from build123d import *

# Parameters (mm, degrees)
F0_W      = 25.4
F0_H      = 25.4
F1_DEPTH  = 27.94
F2_R      = 5.08
F3_R      = 5.08
F4_R      = 5.08
F5_R      = 5.08
F6_W      = 15.24
F6_H      = 7.62
F7_DEPTH  = 12.7
F8_R      = 2.54
F9_R      = 2.54
F10_R     = 2.54
F11_R     = 2.54
F12_R     = 3.175
F14_DEPTH = 9.525


with BuildPart() as f1:
    # F0 (on Front) → F1 (new body)
    with BuildSketch(Plane.XZ):
        with Locations((12.7, -12.7)):
            Rectangle(F0_W, F0_H)
    extrude(amount=F1_DEPTH)

    # F2
    f2_edges = [f1.edges().sort_by_distance(p)[0] for p in [
        (25.4, -13.97, 0),
    ]]
    fillet(f2_edges, radius=F2_R)

    # F3
    f3_edges = [f1.edges().sort_by_distance(p)[0] for p in [
        (0, -13.97, 0),
    ]]
    fillet(f3_edges, radius=F3_R)

    # F4
    f4_edges = [f1.edges().sort_by_distance(p)[0] for p in [
        (25.4, -13.97, -25.4),
    ]]
    fillet(f4_edges, radius=F4_R)

    # F5
    f5_edges = [f1.edges().sort_by_distance(p)[0] for p in [
        (0, -13.97, -25.4),
    ]]
    fillet(f5_edges, radius=F5_R)

    # F6 (on face) → F7 (join)
    with BuildSketch(Plane(origin=(0, 0, 0), x_dir=(-1, 0, 0), z_dir=(0, 1, 0))):
        with Locations((-12.7, -8.89)):
            Rectangle(F6_W, F6_H)
    extrude(amount=F7_DEPTH)

    # F8
    f8_edges = [f1.edges().sort_by_distance(p)[0] for p in [
        (5.08, 6.35, -5.08),
    ]]
    fillet(f8_edges, radius=F8_R)

    # F9
    f9_edges = [f1.edges().sort_by_distance(p)[0] for p in [
        (5.08, 6.35, -12.7),
    ]]
    fillet(f9_edges, radius=F9_R)

    # F10
    f10_edges = [f1.edges().sort_by_distance(p)[0] for p in [
        (20.32, 6.35, -5.08),
    ]]
    fillet(f10_edges, radius=F10_R)

    # F11
    f11_edges = [f1.edges().sort_by_distance(p)[0] for p in [
        (20.32, 6.35, -12.7),
    ]]
    fillet(f11_edges, radius=F11_R)

    # F12 (on face) → F14 (join)
    with BuildSketch(Plane(origin=(0, 12.7, 0), x_dir=(-1, 0, 0), z_dir=(0, 1, 0))):
        with Locations((-12.7, -8.89)):
            Circle(F12_R)
    extrude(amount=F14_DEPTH)


solid = f1.part
Model file for the job. Use its own axes, mm. A direction names the side the tool comes from. Give positions to 0.01 mm unless a question says otherwise; leave off trailing zeros. Order: outer loops, then holes, each group sorted by start corner. A loop starts at its lowest first (then second) coordinate and runs counter-clockwise, first axis right, second up. Notation, with made-up numbers: (78.25, 74) -> (85.25, 74) arc R9 cw to (85.25, 79) -> close; hole circle Ø3 at (-3, 12.5). An arc over 180 degrees is marked (long way). Use CSV: the item, a comma, the result in double quotes.
1. Band-saw the part on C-C, the plane x = 12. Give the cut face in (y, z) (3 decimals).
Outcome:
outline,"(-27.94, -25.4) -> (0, -25.4) -> (0, -12.7) -> (12.7, -12.7) -> (12.7, -11.987) -> (22.225, -11.987) -> (22.225, -5.793) -> (12.7, -5.793) -> (12.7, -5.08) -> (0, -5.08) -> (0, 0) -> (-27.94, 0) -> close"
2. Drill centre lines: line 1 along Y through (x, z) = (9.75, -22.25); line 2 along X through (y, z) = (1.5, -7.5); line 3 along Y through (x, z) = (7.25, -9). Where is each one in solid material? Low to high. Write a range as from..to.
Outcome:
line 1,"-27.94..0"
line 2,"5.08..20.32"
line 3,"-27.94..12.7"
3. Drop flat-ended pins along their axis: pin 1 (10 mm diameter, centred on y = 10.5, z = -6.5, fed in from -X); pin 2 (5 mm diameter, centred on x = 10.5, y = 9.5, fed in from +Z); pin 3 (8 mm diameter, centred on x = 12.5, y = 5.5, fed in from -Z). Give the stop position or say it passes through.
Outcome:
pin 1,"x = 5.08"
pin 2,"z = -5.08"
pin 3,"z = -12.7"
4. Band-saw the part on A-A, the plane y = 2. Give the cut face in (x, z), then the cut area to 3 significant figures.
Outcome:
outline,"(5.08, -10.16) arc R2.54 ccw to (7.62, -12.7) -> (17.78, -12.7) arc R2.54 ccw to (20.32, -10.16) -> (20.32, -7.62) arc R2.54 ccw to (17.78, -5.08) -> (7.62, -5.08) arc R2.54 ccw to (5.08, -7.62) -> close"
area,"111 mm²"
5. Band-saw the part on D-D, the plane x = 6.25. Give the cut face in (y, z), then the cut area to 3 significant figures.
Outcome:
outline,"(-27.94, -25.4) -> (0, -25.4) -> (0, -12.3) -> (12.7, -12.3) -> (12.7, -5.48) -> (0, -5.48) -> (0, 0) -> (-27.94, 0) -> close"
area,"796 mm²"
6. 3-axis set-ups, long thin cutter, end or side, ignore diameter. For faces 1 (the cylindrical face through (19.556, 6.439, -5.804)), 2 (the flat face through (13, 6, -12.7)), 3 (the flat face through (13, 6, -5.08)), 4 (the flat face through (20.32, 6, -9)), 5 (the flat face through (5.08, 6, -9)): which of +Z, -Z, +X, -X, +Y, -Y reach the whole face in a straight line?
Outcome:
face 1,"+Z, +X, +Y"
face 2,"-Z, +X, -X, +Y"
face 3,"+Z, +X, -X, +Y"
face 4,"+Z, -Z, +X, +Y"
face 5,"+Z, -Z, -X, +Y"
7. Band-saw the part on B-B, the plane z = -8.89. Give the cut face in (x, y) (3 decimals), then the cut area to 3 significant figures.
Outcome:
outline,"(0, -27.94) -> (25.4, -27.94) -> (25.4, 0) -> (20.32, 0) -> (20.32, 12.7) -> (15.875, 12.7) -> (15.875, 22.225) -> (9.525, 22.225) -> (9.525, 12.7) -> (5.08, 12.7) -> (5.08, 0) -> (0, 0) -> close"
area,"964 mm²"
